Design review of the part built by this model. Coordinates are the model's own, in mm. A direction names the side the tool comes from. Give positions to 0.01 mm unless a question says otherwise; leave off trailing zeros. Loops run counter-clockwise (first coordinate to the right, second up) from the corner with the lowest first, then second, coordinate; pieces in that order, holes last. Notation, with made-up numbers: (-28, 7) -> (-23, 7) arc R33 cw to (-23, 39) -> close; hole circle Ø6 at (83.25, -27). An arc over 180 degrees is marked (long way). Use a Markdown table: item, result. Add a question column.
1. Add section B-B (x = 0). State the section outline as (y, z) points, and give its area (3 significant figures).
2. Draft analysis for pull direction X (two halves, no side actions). For faces 1 (the cylindrical face through (-8, 5.14, 6.89)), 2 (the flat face through (2, 0, 0)), state which applies: pulls with the +X half, pulls with the -X half, needs draft (parallel to the pull), parting line crosses it, or undercut.
3. Add section A-A (z = 9.5). Count the separate pieces of the cut face and the enclosed holes in it, and give its area (3 significant figures).
4. For faces 3 (the flat face through (-7, -1, 10.9)), 4 (the cylindrical face through (-4.964, 5.37, 6.895)), list the 3-axis set-ups (+Z, -Z, +X, -X, +Y, -Y) from which the entire face can be reached by the end or side of a thin tool; tool diameter is ignored.
5. Add section D-D (y = -3.75). State the section outline as (x, z) points, and give its area (3 significant figures).
6. To check wall thickness, follow line 1 (Y direction, x = 0, z = 1.6); line 2 (X direction, y = -2, z = 4.5); line 3 (Y direction, x = 0, z = 0.1). State the ranges of each line that lie inside material, in increasing order.
7. For pin 1 Ø4 at (x, y) = (0.5, -0.5) entering from +Z; pin 2 Ø5 at (x, z) = (-4.5, 4) entering from -Y, all flat-tipped, find the tip position at first contact; note any pin that passes through.
```python
from build123d import *

# Parameters (mm, degrees)
SKETCH_1_R               = 10.4
EXTRUDE_1_DEPTH          = 3
SKETCH_3_R               = 2.4
SKETCH_3_R_2             = 0.75
EXTRUDE_3_DEPTH          = 7.9
PATTERN_CIRCULAR_1_COUNT = 6
SKETCH_4_R               = 0.75
CUT_EXTRUDE_1_DEPTH      = 17.695208894
PATTERN_CIRCULAR_2_COUNT = 3
SKETCH_5_R               = 1.1
CUT_EXTRUDE_2_DEPTH      = 17.695208894
SKETCH_5_4_R             = 2.55
SKETCH_5_4_R_2           = 1.1
CUT_EXTRUDE_3_DEPTH      = 2.6


with BuildPart() as part:
    # Sketch 1 → Extrude 1 (new body)
    with BuildSketch(Plane.XY):
        Circle(SKETCH_1_R)
    extrude(amount=EXTRUDE_1_DEPTH)

    # Sketch 3 → Extrude 3 (add)
    with BuildSketch(Plane.XY.offset(3)):
        with Locations(Location((-5.656854249, 5.656854249, 0), (0, 0, 135))):
            Circle(SKETCH_3_R)
        with Locations((-5.656854249, 5.656854249)):
            Circle(SKETCH_3_R_2, mode=Mode.SUBTRACT)
    extrude_3 = extrude(amount=EXTRUDE_3_DEPTH)

    # Pattern Circular 1: Extrude 3 ×6 about axis
    pattern_circular_1_axis = Axis((0, 0, 0), (0, 0, 1))
    for i in range(1, PATTERN_CIRCULAR_1_COUNT):
        add(extrude_3.rotate(pattern_circular_1_axis, i * 360 / PATTERN_CIRCULAR_1_COUNT))

    # Sketch 4 → Cut-Extrude 1 (cut, through all)
    with BuildSketch(Plane.XY.offset(3)):
        with Locations((-1.793150944, 6.69213043)):
            Circle(SKETCH_4_R)
    cut_extrude_1 = extrude(amount=-CUT_EXTRUDE_1_DEPTH, mode=Mode.SUBTRACT)

    # Pattern Circular 2: Cut-Extrude 1 ×3 about axis
    pattern_circular_2_axis = Axis((0, 0, 0), (0, 0, 1))
    for i in range(1, PATTERN_CIRCULAR_2_COUNT):
        add(cut_extrude_1.rotate(pattern_circular_2_axis, i * 360 / PATTERN_CIRCULAR_2_COUNT), mode=Mode.SUBTRACT)

    # Sketch 5 → Cut-Extrude 2 (cut, through all)
    with BuildSketch(Plane.XY.offset(3)):
        Circle(SKETCH_5_R)
    extrude(amount=-CUT_EXTRUDE_2_DEPTH, mode=Mode.SUBTRACT)

    # Sketch 5_4 → Cut-Extrude 3 (cut)
    with BuildSketch(Plane.XY.offset(3)):
        Circle(SKETCH_5_4_R)
        Circle(SKETCH_5_4_R_2, mode=Mode.SUBTRACT)
    extrude(amount=-CUT_EXTRUDE_3_DEPTH, mode=Mode.SUBTRACT)


solid = part.part
```
Taken from the geometry:
| question | item | result |
|---|---|---|
| 1 | outline | (-10.4, 0) -> (-1.1, 0) -> (-1.1, 0.4) -> (-2.55, 0.4) -> (-2.55, 3) -> (-6.51, 3) -> (-6.51, 10.9) -> (-8.94, 10.9) -> (-8.94, 3) -> (-10.4, 3) -> close; (1.1, 0) -> (10.4, 0) -> (10.4, 3) -> (8.94, 3) -> (8.94, 10.9) -> (6.51, 10.9) -> (6.51, 3) -> (2.55, 3) -> (2.55, 0.4) -> (1.1, 0.4) -> close |
| 1 | area | 86.6 mm^2 |
| 2 | face 1 | undercut |
| 2 | face 2 | needs draft |
| 3 | separate pieces | 6 |
| 3 | enclosed holes | 6 |
| 3 | area | 98.0 mm^2 |
| 4 | face 3 | +Z, +X, -X, +Y, -Y |
| 4 | face 4 | +Z |
| 5 | outline | (-9.7, 0) -> (9.7, 0) -> (9.7, 3) -> (7.11, 3) -> (7.11, 10.9) -> (4.2, 10.9) -> (4.2, 3) -> (-6.01, 3) -> (-6.01, 10.9) -> (-9.44, 10.9) -> (-9.44, 3) -> (-9.7, 3) -> close |
| 5 | area | 108 mm^2 |
| 6 | line 1 | y = -10.4 to -2.55, 2.55 to 10.4 |
| 6 | line 2 | x = -10.13 to -8.47, -6.98 to -5.33 |
| 6 | line 3 | y = -10.4 to -1.1, 1.1 to 10.4 |
| 7 | pin 1 | stops at z = 3 |
| 7 | pin 2 | stops at y = -10.16 |
